from build123d import *

# Parameters (mm, degrees)
EXTRUDE_1_DEPTH = 3
SKETCH_3_W      = 60
SKETCH_3_H      = 10
EXTRUDE_3_DEPTH = 3
EXTRUDE_4_DEPTH = 3
EXTRUDE_5_DEPTH = 3
FILLET_1_R      = 1.5
FILLET_2_R      = 1.5
M4X0_71_D       = 3.3


with BuildPart() as part:
    # Sketch 1 → Extrude 1 (new body)
    with BuildSketch(Plane(origin=(0, 0, 0), x_dir=(1, 0, 0), z_dir=(0, 1, 0))):
        with BuildLine():
            Line((8.241767279, 0), (101.758232721, 0))
            ThreePointArc((101.758232721, 0), (110, 27.5), (101.758232721, 55))
            Line((101.758232721, 55), (8.241767279, 55))
            ThreePointArc((8.241767279, 55), (0, 27.5), (8.241767279, 0))
        make_face()
        with BuildLine():
            Line((9.890774129, 3), (100.109225871, 3))
            ThreePointArc((100.109225871, 3), (107, 27.5), (100.109225871, 52))
            Line((100.109225871, 52), (9.890774129, 52))
            ThreePointArc((9.890774129, 52), (3, 27.5), (9.890774129, 3))
        make_face(mode=Mode.SUBTRACT)
    extrude(amount=EXTRUDE_1_DEPTH)

    # Sketch 4 → Extrude 4 (add, through all)
    with BuildSketch(Plane.XZ):
        with BuildLine():
            Line((27.611432525, -3), (23.02885683, -3))
            ThreePointArc((23.02885683, -3), (25.02885683, -5), (23.02885683, -7))
            Line((23.02885683, -7), (11.02885683, -7))
            ThreePointArc((11.02885683, -7), (9.296806041, -6.000000032), (9.296805985, -4.000000064))
            ThreePointArc((9.296805985, -4.000000064), (8.176529623, -6.057114801), (7.160134889, -8.167489628))
            ThreePointArc((7.160134889, -8.167489628), (8.888465293, -9.51870823), (11.02885683, -10))
            Line((11.02885683, -10), (23.02885683, -10))
            ThreePointArc((23.02885683, -10), (27.212156962, -7.738612788), (27.611432525, -3))
        make_face()
        with BuildLine():
            ThreePointArc((9.296805985, -4.000000064), (10.028856798, -3.267949211), (11.02885683, -3))
            Line((11.02885683, -3), (9.890774129, -3))
            ThreePointArc((9.890774129, -3), (9.590696591, -3.498162612), (9.296805985, -4.000000064))
        make_face()
        with BuildLine():
            Line((86.97114317, -3), (82.388567475, -3))
            ThreePointArc((82.388567475, -3), (82.787843038, -7.738612788), (86.97114317, -10))
            Line((86.97114317, -10), (98.97114317, -10))
            ThreePointArc((98.97114317, -10), (101.111534707, -9.51870823), (102.839865111, -8.167489628))
            ThreePointArc((102.839865111, -8.167489628), (101.823470359, -6.057114766), (100.703193976, -3.999999997))
            ThreePointArc((100.703193976, -3.999999997), (100.703193979, -5.999999998), (98.97114317, -7))
            Line((98.97114317, -7), (86.97114317, -7))
            ThreePointArc((86.97114317, -7), (84.97114317, -5), (86.97114317, -3))
        make_face()
        with BuildLine():
            Line((100.109225871, -3), (98.97114317, -3))
            ThreePointArc((98.97114317, -3), (99.971143169, -3.267949191), (100.703193976, -3.999999997))
            ThreePointArc((100.703193976, -3.999999997), (100.409303389, -3.498162579), (100.109225871, -3))
        make_face()
        with BuildLine():
            ThreePointArc((100.703194034, -50.999999903), (101.823470385, -48.942885182), (102.839865111, -46.832510372))
            ThreePointArc((102.839865111, -46.832510372), (101.111534707, -45.48129177), (98.97114317, -45))
            Line((98.97114317, -45), (86.97114317, -45))
            ThreePointArc((86.97114317, -45), (82.787843038, -47.261387212), (82.388567475, -52))
            Line((82.388567475, -52), (86.97114317, -52))
            ThreePointArc((86.97114317, -52), (84.97114317, -50), (86.97114317, -48))
            Line((86.97114317, -48), (98.97114317, -48))
            ThreePointArc((98.97114317, -48), (100.70319395, -48.999999951), (100.703194034, -50.999999903))
        make_face()
        with BuildLine():
            ThreePointArc((100.109225871, -52), (100.409303419, -51.501837371), (100.703194034, -50.999999903))
            ThreePointArc((100.703194034, -50.999999903), (99.971143219, -51.732050779), (98.97114317, -52))
            Line((98.97114317, -52), (100.109225871, -52))
        make_face()
        with BuildLine():
            ThreePointArc((11.02885683, -45), (8.888465293, -45.48129177), (7.160134889, -46.832510372))
            ThreePointArc((7.160134889, -46.832510372), (8.17652965, -48.942885251), (9.296806044, -51.000000038))
            ThreePointArc((9.296806044, -51.000000038), (9.296806011, -49.000000019), (11.02885683, -48))
            Line((11.02885683, -48), (23.02885683, -48))
            ThreePointArc((23.02885683, -48), (25.02885683, -50), (23.02885683, -52))
            Line((23.02885683, -52), (27.611432525, -52))
            ThreePointArc((27.611432525, -52), (27.212156962, -47.261387212), (23.02885683, -45))
            Line((23.02885683, -45), (11.02885683, -45))
        make_face()
        with BuildLine():
            ThreePointArc((11.02885683, -52), (10.028856848, -51.732050818), (9.296806044, -51.000000038))
            ThreePointArc((9.296806044, -51.000000038), (9.590696621, -51.501837438), (9.890774129, -52))
            Line((9.890774129, -52), (11.02885683, -52))
        make_face()
    extrude(amount=-EXTRUDE_4_DEPTH)



with BuildPart() as body_2:
    # Sketch 3 → Extrude 3 (new body, through all)
    with BuildSketch(Plane.XZ):
        with Locations((55, -27.5)):
            Rectangle(SKETCH_3_W, SKETCH_3_H)
    extrude(amount=-EXTRUDE_3_DEPTH)


with BuildPart() as part_1:
    add(part.part)

    add(body_2.part)  # Extrude 5 merges body 2
    # Sketch 5 → Extrude 5 (add, through all)
    with BuildSketch(Plane.XZ):
        Polygon((27.394984288, -22.5), (8.099598255, -6.998127159), (6.220671523, -9.336852098), (25, -24.424125375), (25, -22.5), align=None)
        Polygon((25, -30.575874625), (6.220671523, -45.663147902), (8.099598255, -48.001872841), (27.394984288, -32.5), (25, -32.5), align=None)
        Polygon((101.900401745, -6.998127159), (82.605015712, -22.5), (85, -22.5), (85, -24.424125375), (103.779328477, -9.336852098), align=None)
        Polygon((82.605015712, -32.5), (101.900401745, -48.001872841), (103.779328477, -45.663147902), (85, -30.575874625), (85, -32.5), align=None)
    extrude(amount=-EXTRUDE_5_DEPTH)

    # Fillet 1
    fillet_1_edges = [part_1.edges().sort_by_distance(p)[0] for p in [
        (11.836069059, 1.5, -45),
        (6.543612581, 1.5, -45.403697731),
        (27.394984288, 1.5, -32.5),
        (25, 1.5, -30.575874625),
        (98.163930941, 1.5, -10),
        (103.456387419, 1.5, -9.596302269),
        (82.605015712, 1.5, -22.5),
        (85, 1.5, -24.424125375),
        (27.394984288, 1.5, -22.5),
        (98.163930941, 1.5, -45),
        (103.456387419, 1.5, -45.403697731),
        (25, 1.5, -24.424125375),
        (82.605015712, 1.5, -32.5),
        (85, 1.5, -30.575874625),
        (11.836069059, 1.5, -10),
        (6.543612581, 1.5, -9.596302269),
        (27.611432525, 1.5, -52),
        (82.388567475, 1.5, -3),
        (27.611432525, 1.5, -3),
        (82.388567475, 1.5, -52),
    ]]
    fillet(fillet_1_edges, radius=FILLET_1_R)

    # Fillet 2
    fillet_2_edges = [part_1.edges().sort_by_distance(p)[0] for p in [
        (8.241767279, 1.5, -55),
        (8.241767279, 1.5, 0),
        (101.758232721, 1.5, 0),
        (101.758232721, 1.5, -55),
    ]]
    fillet(fillet_2_edges, radius=FILLET_2_R)

    # M4x0.71 (through all)
    with Locations(Plane(origin=(-0.1210586, 0, 3.198200318), x_dir=(-1, 0, 0), z_dir=(0, -1, 0))):
        with Locations((-80.8710586, 30.698200318), (-29.3710586, 30.698200318)):
            Hole(M4X0_71_D / 2)


solid = part_1.part
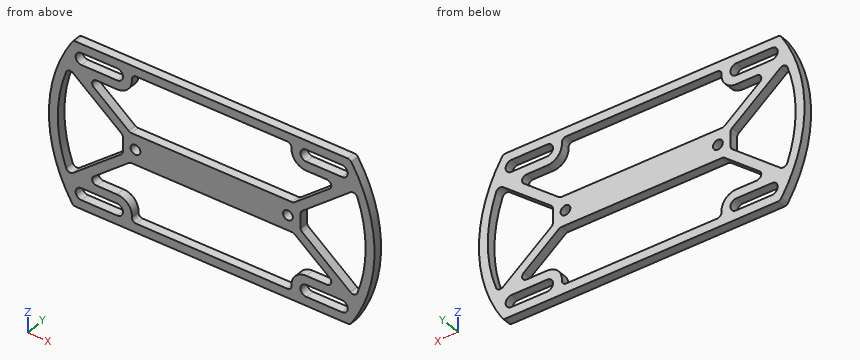
CAD build for the part. Positions are in the model's coordinates, mm. Round coordinates to 2 decimals unless told otherwise and drop trailing zeros. Order: outer loops, then holes, each group sorted by start corner. A loop starts at its lowest first (then second) coordinate and runs counter-clockwise, first axis right, second up. Notation, with made-up numbers: (74, -2) - (85, -2) arc R16 cw to (85, 20) - close; hole circle Ø9 at (51, -24). An arc over 180 degrees is marked (long way). Return JSON: item names as keys, results as strings.
(1) Cut at D-D (y = 1.9). State how many separate pieces and enclosed holes the cut face has, then the cut area to 3 significant figures.
Answer key:
{"separate pieces": "1", "enclosed holes": "10", "area": "2,030 mm^2"}
(2) Cut at A-A (z = -27.5). Give the cut face in (x, y).
Answer key:
{"outline": "(0, 0) - (3, 0) - (3, 3) - (0, 3) - close; (25, 0) - (27.6, 0) - (27.6, 3) - (25, 3) - close; (30.9, 0) - (79.1, 0) - (79.1, 3) - (30.9, 3) - close; (82.4, 0) - (85, 0) - (85, 3) - (82.4, 3) - close; (107, 0) - (110, 0) - (110, 3) - (107, 3) - close"}
(3) Cut at C-C (z = -39). Give the cut face in (x, y).
Answer key:
{"outline": "(1.34, 0) - (4.43, 0) - (4.43, 3) - (1.34, 3) - close; (14.51, 0) - (19.3, 0) - (19.3, 3) - (14.51, 3) - close; (90.7, 0) - (95.49, 0) - (95.49, 3) - (90.7, 3) - close; (105.57, 0) - (108.66, 0) - (108.66, 3) - (105.57, 3) - close"}
(4) Cut at B-B (x = 89.5). Give the cut face in (y, z).
Answer key:
{"outline": "(0, -55) - (3, -55) - (3, -52) - (0, -52) - close; (0, -48) - (3, -48) - (3, -45) - (0, -45) - close; (0, -38.04) - (3, -38.04) - (3, -34.19) - (0, -34.19) - close; (0, -20.81) - (3, -20.81) - (3, -16.96) - (0, -16.96) - close; (0, -10) - (3, -10) - (3, -7) - (0, -7) - close; (0, -3) - (3, -3) - (3, 0) - (0, 0) - close"}
(5) Wall check: probe 1 along Z at (x, y) = (29.25, 1.05); probe 2 along Z at (x, y) = (73.5, 1.65); probe 3 along X at (y, z) = (1.65, -27). Give the ranges that are in metal, low to high. Write a range as from..to.
Answer key:
{"probe 1": "z = -55..-51.98, -32.5..-29.15, -25.85..-22.5, -3.02..0", "probe 2": "z = -55..-52, -32.5..-22.5, -3..0", "probe 3": "x = 0..3, 25..27.68, 30.82..79.18, 82.32..85, 107..110"}
